Part print with two shaded views. Sizes in mm from the minimum x, y, z corner. Coordinates: 2 decimals unless noted, no trailing zeros. Loops run counter-clockwise (first coordinate to the right, second up) from the corner with the lowest first, then second, coordinate; pieces in that order, holes last. Notation, with made-up numbers: M -23,57.5 L -9,57.5 A25 ccw -9,92.5 Z; hole C 32.5,58.5 d10. An arc over 180 degrees is marked long. Write item = value, one per line. Start each with the question number.
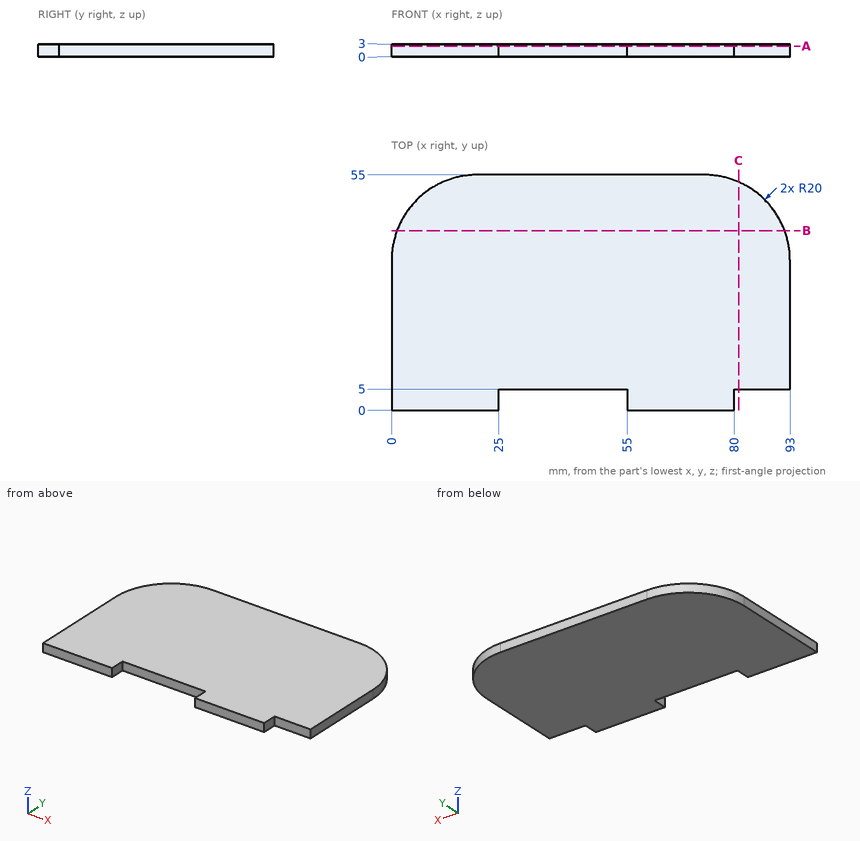
Item 1: Cut at B-B (y = 42). Give the cut face in (x, z) (3 decimals), plus the area to 3 significant figures.
Item 2: Cut at C-C (x = 81). Give the cut face in (y, z), plus the area to 3 significant figures.
Item 3: Pin check, flat tips, straight feed: pin 1 Ø5 at (x, y) = (83, 43) entering from -Z; pin 2 Ø0.9 at (x, z) = (87, 2) entering from -Y; pin 3 Ø1 at (x, z) = (14, 1) entering from +Y; pin 4 Ø1.5 at (y, z) = (2.5, 1) entering from +X. Stop position of each tip, or through.
Item 4: Cut at A-A (z = 2.5). Give the cut face in (x, y), plus the area to 3 significant figures.
Item 5: Probe L1, parallel to Y at x = 46, z = 1.7; L2, parallel to X at y = 4.5, z = 1.85; L3, parallel to X at y = 46.5, z = 2.7. List the from-to ranges inside material, lowest first.
Reported:
q1.outline = M 1.265,0 L 91.735,0 L 91.735,3 L 1.265,3 Z
q1.area = 271 mm^2
q2.outline = M 5,0 L 53.33,0 L 53.33,3 L 5,3 Z
q2.area = 145 mm^2
q3.pin_1 = 0
q3.pin_2 = 5
q3.pin_3 = 54.23
q3.pin_4 = 80
q4.outline = M 0,0 L 25,0 L 25,5 L 55,5 L 55,0 L 80,0 L 80,5 L 93,5 L 93,35 A20 ccw 73,55 L 20,55 A20 ccw 0,35 Z
q4.area = 4,730 mm^2
q5.L1 = 5 to 55
q5.L2 = 0 to 25, 55 to 80
q5.L3 = 3.64 to 89.36
